Design review of the part shown in the three views and the two pictorial views. Dimensions are in mm from the part's minimum x, y and z. A direction names the side the tool comes from. Coordinates: 2 decimals unless noted, no trailing zeros. Order: outer loops, then holes, each group sorted by start corner. A loop starts at its lowest first (then second) coordinate and runs counter-clockwise, first axis right, second up. Notation, with made-up numbers: (1.5, 58) -> (51.5, 58) arc R19 ccw to (51.5, 70) -> close; hole circle Ø4 at (1.5, 12). An arc over 180 degrees is marked (long way). Write item = value, one per line. Start each with the question number.
1) Consider section D-D on y = 32.5. Give the boundary of the cut face in (x, z), and give its area (4 significant figures).
2) Machinability: for the marked faces 1 and 2, which of the approach directions +Z, -Z, +X, -X, +Y, -Y give a long, thin tool a straight path to every point of the face, cutting with its end or side? Answer none if there is none.
3) Wall thickness on probe 1 along Z at (x, y) = (55.5, 23); probe 2 along X at (y, z) = (46, 12); probe 3 along Y at (x, z) = (29, 28) (1 decimal): over which ranges is each line inside the solid? List them lowest first. Write a range as [from, to].
4) Consider section C-C on z = 37.5. Give the boundary of the cut face in (x, y) (1 decimal), and give its area (3 significant figures).
5) Insertion check: pin 1 Ø10 at (x, y) = (24.5, 63.5) entering from +Z; pin 2 Ø4 at (x, y) = (81.47, 46.52) entering from +Z; pin 3 Ø10 at (x, z) = (46, 42.5) entering from -Y (1 decimal). Each pin has a flat end and moves straight along its axis. Give the tip position at first contact, or say it passes through.
6) Consider section B-B on x = 100. Give the boundary of the cut face in (y, z).
7) Consider section A-A on y = 18. Give the boundary of the cut face in (x, z) (1 decimal), and give its area (3 significant figures).
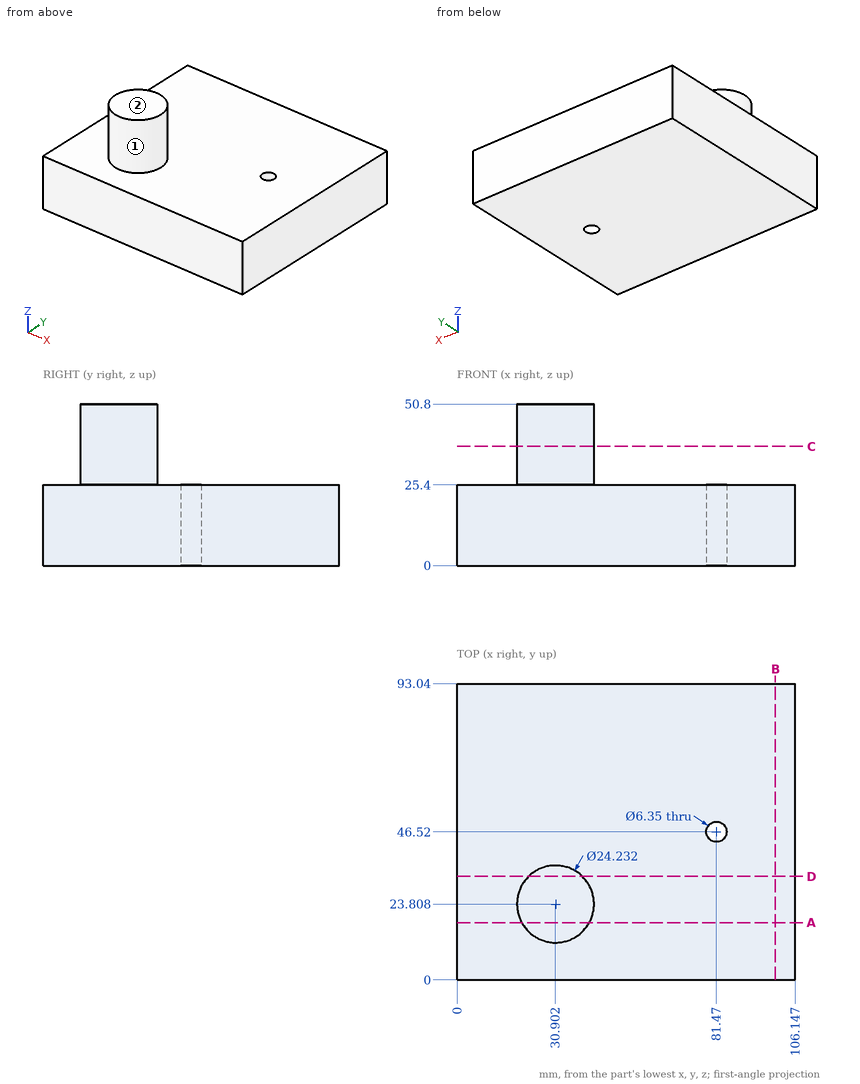
Answer sheet:
q1.outline = (0, 0) -> (106.15, 0) -> (106.15, 25.4) -> (39.34, 25.4) -> (39.34, 50.8) -> (22.46, 50.8) -> (22.46, 25.4) -> (0, 25.4) -> close
q1.area = 3,125 mm2
q2.face_1 = +Z
q2.face_2 = +Z, +X, -X, +Y, -Y
q3.probe_1 = [0, 25.4]
q3.probe_2 = [0, 78.34], [84.6, 106.15]
q3.probe_3 = [11.8, 35.8]
q4.outline = circle Ø24.2 at (30.9, 23.8)
q4.area = 461 mm2
q5.pin_1 = 25.4
q5.pin_2 = through
q5.pin_3 = 17.1
q6.outline = (0, 0) -> (93.04, 0) -> (93.04, 25.4) -> (0, 25.4) -> close
q7.outline = (0, 0) -> (106.1, 0) -> (106.1, 25.4) -> (41.5, 25.4) -> (41.5, 50.8) -> (20.3, 50.8) -> (20.3, 25.4) -> (0, 25.4) -> close
q7.area = 3,240 mm2
